For this review, take the finished solid that the model builds, in its own axes (mm). A direction names the side the tool comes from. Give positions to 0.01 mm unless a question says otherwise; leave off trailing zeros. Order: outer loops, then holes, each group sorted by start corner. A loop starts at its lowest first (then second) coordinate and runs counter-clockwise, first axis right, second up. Notation, with made-up numbers: (-29, 35.5) -> (25, 35.5) arc R23 ccw to (25, 72.5) -> close; hole circle Ø3 at (73, 67). An arc over 180 degrees is marked (long way). Return JSON: item names as keys, results as strings. Group by question number.
1) Add section D-D (x = 7.75). Give the boundary of the cut face in (y, z), then the cut area to 3 significant figures.
2) Insertion check: P1, Ø3, axis at x = -9, z = 2.5, coming from the -Y side; P2, Ø3, axis at x = 10, z = 3, coming from the +Y side; P3, Ø5, axis at x = 15.5, y = 20, coming from the +Z side; P4, Ø2.5, axis at x = 7.75, y = 33.42, coming from the +Z side. Each pin has a flat end and moves straight along its axis. Give the tip position at first contact, or say it passes through.
3) To check wall thickness, follow line 1 along X through (y, z) = (-2.5, 4.6); line 2 along Y through (x, z) = (-7.75, 4.5); line 3 along Y through (x, z) = (6.5, 5.1). State the ranges of each line that lie inside material, in increasing order.
4) For faces 4 (the face through (8, 52, 3)), 5 (the face through (12, -3, 3)), 6 (the face through (6.05, 20, 3)), list the 3-axis set-ups (+Z, -Z, +X, -X, +Y, -Y) from which the entire face can be reached by the end or side of a thin tool; tool diameter is ignored.
5) Add section B-B (y = -1). Give the boundary of the cut face in (x, z), then the cut area to 3 significant figures.
6) Add section A-A (y = 20). Give the boundary of the cut face in (x, z).
7) Add section C-C (x = 15). Give the boundary of the cut face in (y, z), then the cut area to 3 significant figures.
8) The part is to be moulded in two halves that separate along Y. For faces 1 (the face through (-16.61, 21.01, 2.96)), 2 (the face through (0, 34, 0)), 3 (the face through (8, 0, 3)), say which applies: released by +Y, released by -Y, zero draft, split by the parting line, or undercut.
from build123d import *

# Parameters (mm, degrees)
ESQUISSE1_R        = 1.5
BOSS_EXTRU_1_DEPTH = 6


with BuildPart() as part:
    # Esquisse1 → Boss.-Extru.1 (new body)
    with BuildSketch(Plane.XY):
        Polygon((-20, 58), (-12, 58), (-12, 52), (-4, 52), (-4, 58), (4, 58), (4, 52), (12, 52), (12, 58), (20, 58), (20, -1), (20, -6), (12, -6), (12, 0), (4, 0), (4, -6), (-4, -6), (-4, 0), (-12, 0), (-12, -6), (-20, -6), align=None)
        with Locations((-15.5, 20)):
            Circle(ESQUISSE1_R, mode=Mode.SUBTRACT)
        with Locations((-7.75, 33.423393759)):
            Circle(ESQUISSE1_R, mode=Mode.SUBTRACT)
        with Locations((7.75, 33.423393759)):
            Circle(ESQUISSE1_R, mode=Mode.SUBTRACT)
        with Locations((15.5, 20)):
            Circle(ESQUISSE1_R, mode=Mode.SUBTRACT)
        with Locations((7.75, 6.576606241)):
            Circle(ESQUISSE1_R, mode=Mode.SUBTRACT)
        with Locations((-7.75, 6.576606241)):
            Circle(ESQUISSE1_R, mode=Mode.SUBTRACT)
        with BuildLine():
            Line((-6.05, 27), (-6.05, 13))
            ThreePointArc((-6.05, 13), (0, 6.95), (6.05, 13))
            Line((6.05, 13), (6.05, 27))
            ThreePointArc((6.05, 27), (0, 33.05), (-6.05, 27))
        make_face(mode=Mode.SUBTRACT)
    extrude(amount=BOSS_EXTRU_1_DEPTH)


solid = part.part
Evaluation:
{
 "1": {"outline": "(0, 0) -> (5.08, 0) -> (5.08, 6) -> (0, 6) -> close; (8.08, 0) -> (31.92, 0) -> (31.92, 6) -> (8.08, 6) -> close; (34.92, 0) -> (52, 0) -> (52, 6) -> (34.92, 6) -> close", "area": "276 mm^2"},
 "2": {"P1": "y = 0", "P2": "y = 52", "P3": "z = 6", "P4": "through"},
 "3": {"line 1": "-20 to -12, -4 to 4, 12 to 20", "line 2": "0 to 5.08, 8.08 to 31.92, 34.92 to 52", "line 3": "0 to 5.75, 7.41 to 32.59, 34.25 to 52"},
 "4": {"face 4": "+Z, -Z, +Y", "face 5": "+Z, -Z, -Y", "face 6": "+Z, -Z"},
 "5": {"outline": "(-20, 0) -> (-12, 0) -> (-12, 6) -> (-20, 6) -> close; (-4, 0) -> (4, 0) -> (4, 6) -> (-4, 6) -> close; (12, 0) -> (20, 0) -> (20, 6) -> (12, 6) -> close", "area": "144 mm^2"},
 "6": {"outline": "(-20, 0) -> (-17, 0) -> (-17, 6) -> (-20, 6) -> close; (-14, 0) -> (-6.05, 0) -> (-6.05, 6) -> (-14, 6) -> close; (6.05, 0) -> (14, 0) -> (14, 6) -> (6.05, 6) -> close; (17, 0) -> (20, 0) -> (20, 6) -> (17, 6) -> close"},
 "7": {"outline": "(-6, 0) -> (18.59, 0) -> (18.59, 6) -> (-6, 6) -> close; (21.41, 0) -> (58, 0) -> (58, 6) -> (21.41, 6) -> close", "area": "367 mm^2"},
 "8": {"face 1": "undercut", "face 2": "zero draft", "face 3": "released by -Y"}
}
